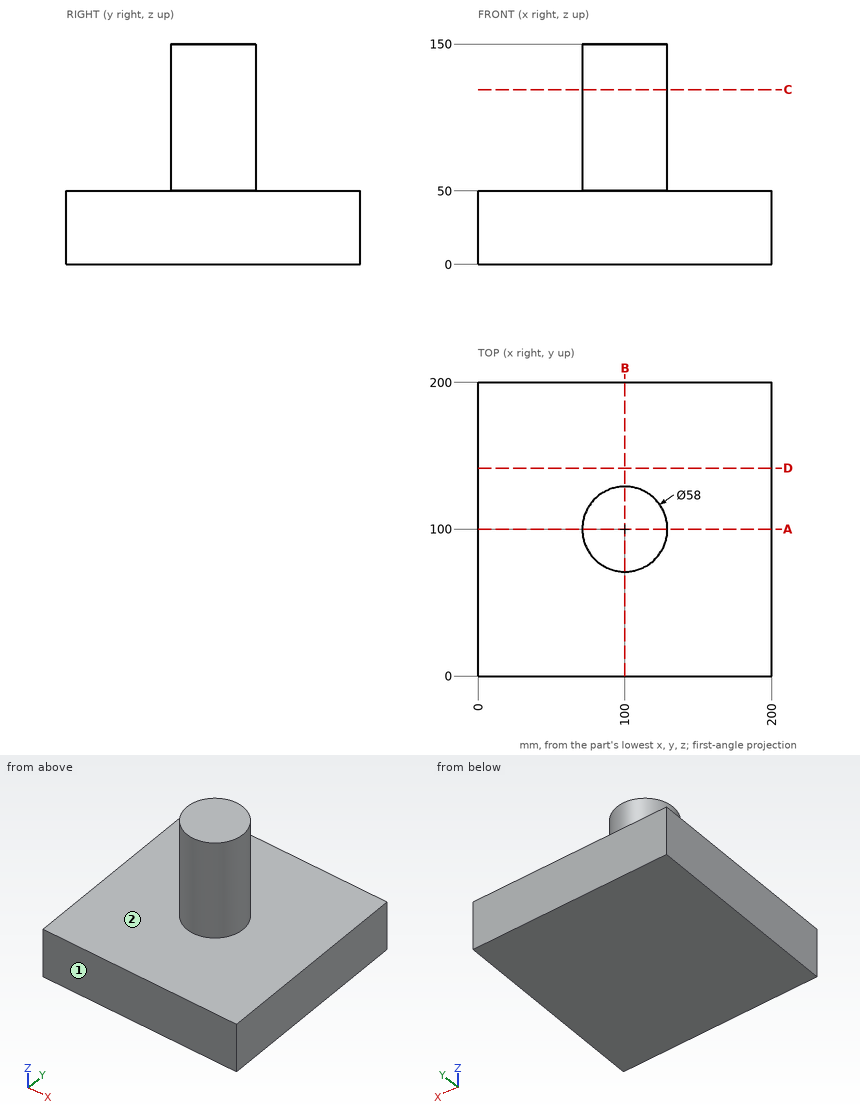
Study the drawing (mm; zero at the part's minimum x, y, z) and answer. A direction names the side the tool comes from. Round coordinates to 2 decimals unless told otherwise and drop trailing zeros. Write each loop counter-clockwise with the first axis right and the second up, starting at its lowest first coordinate (ties: lowest second). Pieces come first, ordered by that corner, then holes.
1) Straight lines are drawn through the part: line 1 (Z direction, x = 42, y = 67); line 2 (X direction, y = 77.5, z = 122); line 3 (Y direction, x = 103.5, z = 57). For each, find the intervals that lie inside material, in ascending order.
2) Given pin 1 Ø3 at (y, z) = (101, 99) entering from +X; pin 2 Ø4 at (x, z) = (128, 109) entering from -Y; pin 3 Ø4 at (x, z) = (100, 111.5) entering from +Y, each flat-ended and moving along its own axis, determine where each tip first touches the part or whether it passes through.
3) A cutting plane is placed at D-D (y = 141.5). Give the vertices of the cut face in (x, z).
4) A tool of negligible diameter and unlimited length cuts with its end or side. For the marked faces 1 and 2, from which of +Z, -Z, +X, -X, +Y, -Y can it reach the whole face along a straight path? Write none if from no direction.
5) A cutting plane is placed at A-A (y = 100). Give the vertices of the cut face in (x, z).
6) A cutting plane is placed at C-C (z = 119). Give the vertices of the cut face in (x, y).
Completed:
1. line 1: z = 0 to 50
1. line 2: x = 81.7 to 118.3
1. line 3: y = 71.21 to 128.79
2. pin 1: stops at x = 129
2. pin 2: stops at y = 87.15
2. pin 3: stops at y = 129
3. outline: (0, 0) - (200, 0) - (200, 50) - (0, 50) - close
4. face 1: +Z, -Z, +X, -X, -Y
4. face 2: +Z
5. outline: (0, 0) - (200, 0) - (200, 50) - (129, 50) - (129, 150) - (71, 150) - (71, 50) - (0, 50) - close
6. outline: circle Ø58 at (100, 100)
